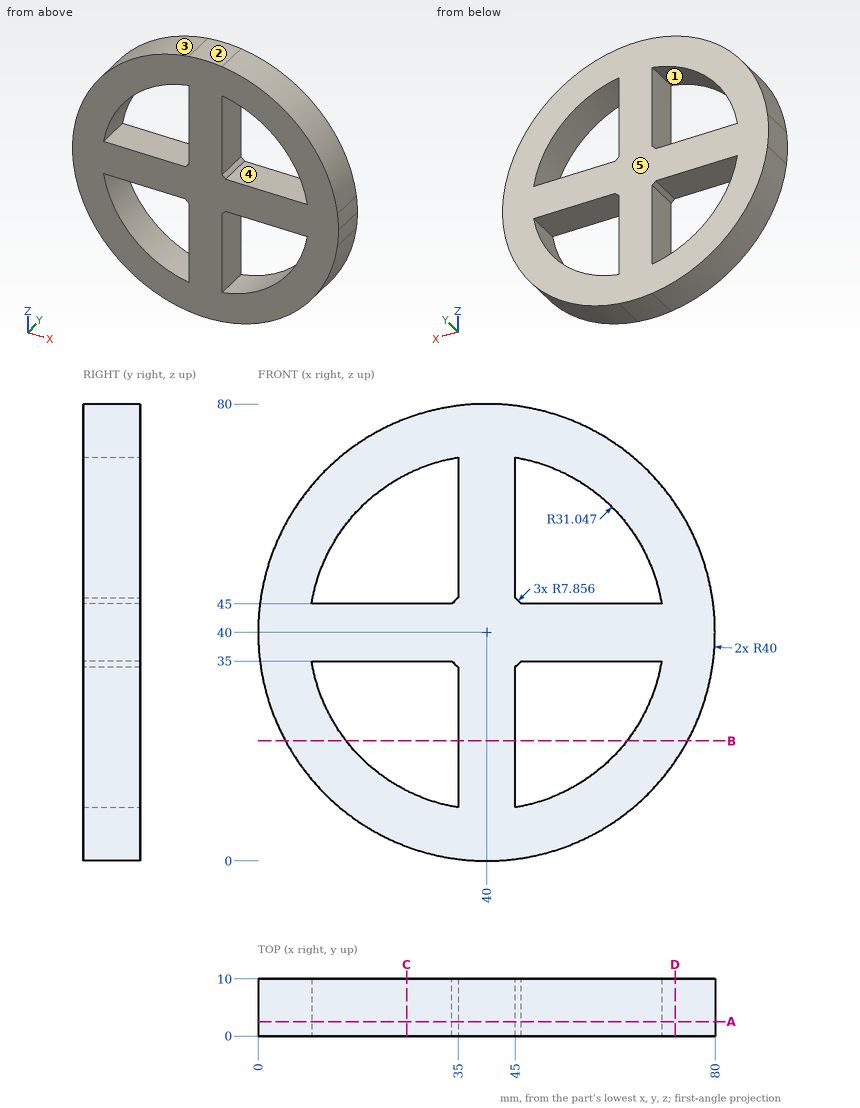
Geometry: see drawing. Coordinates: mm, zero at the bounding-box minimum. A direction names the side the tool comes from. Coordinates: 2 decimals unless noted, no trailing zeros. Loops run counter-clockwise (first coordinate to the right, second up) from the corner with the lowest first, then second, coordinate; pieces in that order, holes last. Notation, with made-up numbers: M 83.25,57 L 135.25,57 A20 cw 135.25,67 Z; hole C 56.5,52.25 d11. An arc over 180 degrees is marked long. Put each result on its own line as item: value. Start each with the question number.
1) Reachability of the marked faces 4 and 5 from +Z, -Z, +X, -X, +Y, -Y: full face, straight path, thin tool, end or side. Return the list, or none.
2) Ray query, L1, parallel to Z at x = 22, y = 1; L2, parallel to X at y = 5.5, z = 66; L3, parallel to X at y = 9.25, z = 26.5. Return the intervals inside material, ascending. Write a range as from..to.
3) Cut plane A-A on y = 2.5. Return the cut outline in (x, z).
4) Contact query for flat-ended pins moving along their axis: pin 1 Ø4 at (x, y) = (63.5, 7.5) entering from +Z; pin 2 Ø3 at (y, z) = (4, 20) entering from +X (1 decimal); pin 3 Ø5 at (x, y) = (40.5, 2.5) entering from -Z; pin 4 Ø2 at (x, z) = (35.5, 68.5) entering from -Y. Output: stop coordinate, or through.
5) Cut plane D-D on x = 73. Return the cut outline in (y, z) (1 decimal).
6) Cut plane B-B on z = 21. Return the cut outline in (x, y) (1 decimal).
7) Pull-direction query (X, two-part tool) for the marked faces 1, 2 and 3; classes: pulls with the +X half, pulls with the -X half, needs draft (parallel to the pull), parting line crosses it, or undercut.
8) Cut plane C-C on x = 26. Return the cut outline in (y, z), then the cut area to 3 significant figures.
The answers:
1. face 4: +Y, -Y
1. face 5: +Z, -Z, +X, -X, +Y
2. L1: z = 4.28..14.7, 35..45, 65.3..75.72
2. L2: x = 9.6..23.03, 35..45, 56.97..70.4
2. L3: x = 2.35..12.04, 35..45, 67.96..77.65
3. outline: M 0.31,35 A40 ccw 35,0.31 A40 ccw 45,0.31 A40 ccw 79.69,35 A40 ccw 80,40 A40 ccw 79.69,45 A40 ccw 45,79.69 A40 ccw 35,79.69 A40 ccw 0.31,45 A40 ccw Z; hole M 9.36,35 A31.05 ccw 35,9.36 L 35,33.94 A7.86 cw 33.94,35 Z; hole M 9.36,45 L 33.94,45 A7.86 cw 35,46.06 L 35,70.64 A31.05 ccw Z; hole M 45,9.36 A31.05 ccw 70.64,35 L 46.06,35 A7.86 cw 45,33.94 Z; hole M 45,46.06 A7.86 cw 46.06,45 L 70.64,45 A31.05 ccw 45,70.64 Z
4. pin 1: stops at z = 73.73
4. pin 2: stops at x = 75.5
4. pin 3: stops at z = 0
4. pin 4: stops at y = 0
5. outline: M 0,17.4 L 10,17.4 L 10,62.6 L 0,62.6 Z
6. outline: M 4.8,0 L 15.4,0 L 15.4,10 L 4.8,10 Z; M 35,0 L 45,0 L 45,10 L 35,10 Z; M 64.6,0 L 75.2,0 L 75.2,10 L 64.6,10 Z
7. face 1: undercut
7. face 2: parting line crosses it
7. face 3: pulls with the -X half
8. outline: M 0,2.53 L 10,2.53 L 10,12.29 L 0,12.29 Z; M 0,35 L 10,35 L 10,45 L 0,45 Z; M 0,67.71 L 10,67.71 L 10,77.47 L 0,77.47 Z
8. area: 295 mm²
